Work out the finished part from the listing and answer in its coordinate system (mm). A direction names the side the tool comes from. Give positions to 0.01 mm unless a question says otherwise; leave off trailing zeros. Loops run counter-clockwise (first coordinate to the right, second up) from the corner with the lowest first, then second, coordinate; pieces in that order, holes last. Notation, with made-up numbers: M -1.75,6.25 L 44.25,6.25 A18 ccw 44.25,17.25 Z; hole C 24,66 d1. An arc over 180 degrees is marked long. Use a Markdown table: item, result.
```python
from build123d import *

# Parameters (mm, degrees)
BOX_W           = 10
BOX_H           = 10
BOX_DEPTH       = 20
PAD_DEPTH       = 0.1
POCKET_DEPTH    = 9
SKETCH_R        = 3.006594
SKETCH_R_2      = 1.465099
SKETCH_R_3      = 2.963699
SKETCH_R_4      = 1.547512
PAD001_DEPTH    = 0.25
SKETCH001_R     = 3.007895
SKETCH001_R_2   = 1.513665
SKETCH001_R_3   = 3.011791
SKETCH001_R_4   = 1.461759
PAD002_DEPTH    = 0.25
SKETCH004_R     = 3.006919
SKETCH004_R_2   = 1.50919
SKETCH004_R_3   = 3.034061
SKETCH004_R_4   = 1.481985
PAD003_DEPTH    = 0.1
SKETCH005_R     = 2.952769
POCKET001_DEPTH = 1


with BuildPart() as part:
    # Box → Box (new body)
    with BuildSketch(Plane.XY):
        with Locations((5, 5)):
            Rectangle(BOX_W, BOX_H)
    extrude(amount=BOX_DEPTH)

    # Sketch002 → Pad (new body)
    with BuildSketch(Plane.XZ):
        with BuildLine():
            ThreePointArc((9.873348, 14.982924), (4.965524, 19.890748), (0.0577, 14.982924))
            Line((0.0577, 14.982924), (0.0577, 0.03838))
            Line((0.0577, 0.03838), (9.873348, 0.03838))
            Line((9.873348, 14.982924), (9.873348, 0.03838))
        make_face()
    extrude(amount=PAD_DEPTH)

    # Sketch003 → Pocket (cut)
    with BuildSketch(Plane.XZ.offset(0.1)):
        with BuildLine():
            ThreePointArc((8.754824, 15.060687), (4.956489, 18.859022), (1.158155, 15.060687))
            Line((1.158155, 15.060687), (1.158155, 1.159242))
            Line((1.158155, 1.159242), (8.754824, 1.159242))
            Line((8.754824, 15.060687), (8.754824, 1.159242))
        make_face()
    extrude(amount=-POCKET_DEPTH, mode=Mode.SUBTRACT)

    # Sketch → Pad001 (new body)
    with BuildSketch(Plane.YZ.offset(10)):
        with Locations((5.000003, 5.047965)):
            Circle(SKETCH_R)
        with Locations((5.000003, 5.047965)):
            Circle(SKETCH_R_2, mode=Mode.SUBTRACT)
        with Locations((5.044216, 15.040468)):
            Circle(SKETCH_R_3)
        with Locations((5.044216, 14.996254)):
            Circle(SKETCH_R_4, mode=Mode.SUBTRACT)
    extrude(amount=PAD001_DEPTH)

    # Sketch001 → Pad002 (new body)
    with BuildSketch(Plane(origin=(0, 0, 0), x_dir=(0, -1, 0), z_dir=(-1, 0, 0))):
        with Locations((-5.044218, 14.996254)):
            Circle(SKETCH001_R)
        with Locations((-5.044218, 14.996254)):
            Circle(SKETCH001_R_2, mode=Mode.SUBTRACT)
        with Locations((-5.000003, 4.959535)):
            Circle(SKETCH001_R_3)
        with Locations((-5.000003, 4.959535)):
            Circle(SKETCH001_R_4, mode=Mode.SUBTRACT)
    extrude(amount=PAD002_DEPTH)

    # Sketch004 → Pad003 (new body)
    with BuildSketch(Plane(origin=(0, 10, 0), x_dir=(-1, 0, 0), z_dir=(0, 1, 0))):
        with Locations((-4.975261, 14.976268)):
            Circle(SKETCH004_R)
        with Locations((-4.975261, 14.976268)):
            Circle(SKETCH004_R_2, mode=Mode.SUBTRACT)
        with Locations((-5.048869, 4.965851)):
            Circle(SKETCH004_R_3)
        with Locations((-5.048869, 4.965851)):
            Circle(SKETCH004_R_4, mode=Mode.SUBTRACT)
    extrude(amount=PAD003_DEPTH)

    # Sketch005 → Pocket001 (cut)
    with BuildSketch(Plane.XY.offset(20)):
        with Locations((5.00277, 4.993419)):
            Circle(SKETCH005_R)
    extrude(amount=-POCKET001_DEPTH, mode=Mode.SUBTRACT)


solid = part.part
```
(1) Consider probe 1 along X at (y, z) = (2, 12); probe 2 along X at (y, z) = (4.25, 12.75); probe 3 along Y at (x, z) = (2.75, 11.25). Determine where each line is inside the solid, lowest interval first. Write a range as [from, to].
Entries:
| item | result |
|---|---|
| probe 1 | x = [0, 1.16], [8.75, 10] |
| probe 2 | x = [-0.25, 1.16], [8.75, 10.25] |
| probe 3 | y = [8.9, 10] |
(2) Which of the six approach directions +Z, -Z, +X, -X, +Y, -Y give full straight-line access (tool end or side, diameter ignored) to faces 1 (the flat face through (1.158, 4, 8)), 2 (the flat face through (0, 5, 5)), 3 (the flat face through (10, 5, 15))?
Entries:
| item | result |
|---|---|
| face 1 | -Y |
| face 2 | -X |
| face 3 | +X |
(3) Given P1, Ø4, axis at y = 4.5, z = 10.5, coming from the +X side; P2, Ø1.5, axis at x = 5, z = 14.5, coming from the +Y side; P3, Ø1.5, axis at x = 3.5, y = 5.5, coming from the +Z side; P4, Ø1.5, axis at y = 5, z = 4.5, coming from the -X side, each flat-ended and moving along its own axis, determine where each tip first touches the part or whether it passes through.
Entries:
| item | result |
|---|---|
| P1 | stops at x = 10.25 |
| P2 | stops at y = 10 |
| P3 | stops at z = 19 |
| P4 | stops at x = 0 |
(4) A cutting plane is placed at B-B (z = 9.5). Write down the section's boundary in (x, y).
Entries:
| item | result |
|---|---|
| outline | M 0,0 L 0.06,0 L 0.06,-0.1 L 1.16,-0.1 L 1.16,8.9 L 8.75,8.9 L 8.75,-0.1 L 9.87,-0.1 L 9.87,0 L 10,0 L 10,10 L 0,10 Z |
(5) The mould has two halves that part along Z. Classify faces 4 (the cylindrical face through (7.82, 5.88, 19.51)), 5 (the flat face through (5, 10, 15)), 6 (the flat face through (5, 5, 0)): released by +Z, released by -Z, zero draft, split by the parting line, or undercut.
Entries:
| item | result |
|---|---|
| face 4 | zero draft |
| face 5 | undercut |
| face 6 | released by -Z |
